The listing builds one solid part. Answer for the finished solid, in the listing's coordinates (mm). Coordinates: 2 decimals unless noted, no trailing zeros. Write each loop counter-clockwise with the first axis right and the second up, starting at its lowest first coordinate (ties: lowest second). Pieces come first, ordered by that corner, then holes.
(1) The part is cut by section A-A on z = 0. Determine the outline of the cut face in (x, y).
(2) The part is cut by section B-B on y = 10. Determine the outline of the cut face in (x, z).
(3) The part is cut by section D-D on y = 31.5. Determine the outline of the cut face in (x, z), plus the area to 3 significant figures.
(4) The part is cut by section C-C on x = 2. Determine the outline of the cut face in (y, z).
(5) Straight lines are drawn through the part: line 1 (Z direction, x = 2.6, y = 3); line 2 (Y direction, x = 1.1, z = -19); line 3 (Y direction, x = 0.65, z = -12.5). For each, find the intervals that lie inside material, in ascending order.
(6) Given P1, Ø4.5, axis at y = 40, z = -19, coming from the -X side, flat-ended and moving along its own axis, determine where the tip first touches the part or whether it passes through.
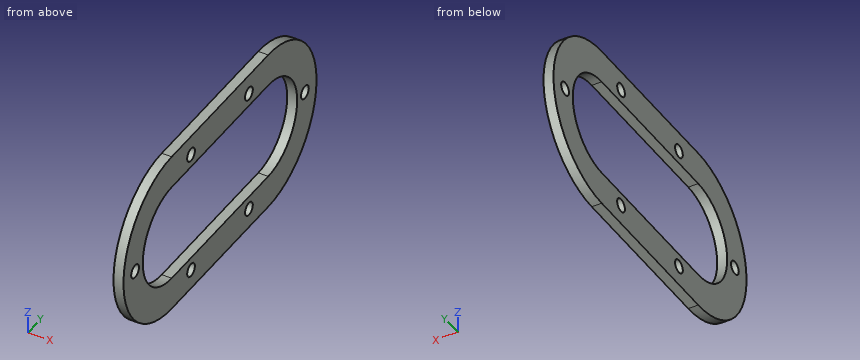
from build123d import *

# Parameters (mm, degrees)
SKETCH1_R           = 2
BOSS_EXTRUDE1_DEPTH = 3


with BuildPart() as part:
    # Sketch1 → Boss-Extrude1 (new body)
    with BuildSketch(Plane.YZ):
        with BuildLine():
            Line((0, 25), (50, 25))
            ThreePointArc((50, 25), (75, 0), (50, -25))
            Line((50, -25), (0, -25))
            ThreePointArc((0, -25), (-25, 0), (0, 25))
        make_face()
        with Locations(Location((10, 19, 0), (0, 0, 270))):
            Circle(SKETCH1_R, mode=Mode.SUBTRACT)
        with Locations(Location((40, 19, 0), (0, 0, 270))):
            Circle(SKETCH1_R, mode=Mode.SUBTRACT)
        with Locations(Location((69, 0, 0), (0, 0, 270))):
            Circle(SKETCH1_R, mode=Mode.SUBTRACT)
        with Locations(Location((-19, 0, 0), (0, 0, 270))):
            Circle(SKETCH1_R, mode=Mode.SUBTRACT)
        with Locations(Location((10, -19, 0), (0, 0, 270))):
            Circle(SKETCH1_R, mode=Mode.SUBTRACT)
        with Locations(Location((40, -19, 0), (0, 0, 270))):
            Circle(SKETCH1_R, mode=Mode.SUBTRACT)
        with BuildLine():
            Line((0, 15), (50, 15))
            ThreePointArc((50, 15), (65, 0), (50, -15))
            Line((50, -15), (0, -15))
            ThreePointArc((0, -15), (-15, 0), (0, 15))
        make_face(mode=Mode.SUBTRACT)
    extrude(amount=BOSS_EXTRUDE1_DEPTH)


solid = part.part
Model answer:
1. outline: (0, -25) - (3, -25) - (3, -21) - (0, -21) - close; (0, -17) - (3, -17) - (3, -15) - (0, -15) - close; (0, 65) - (3, 65) - (3, 67) - (0, 67) - close; (0, 71) - (3, 71) - (3, 75) - (0, 75) - close
2. outline: (0, -25) - (3, -25) - (3, -21) - (0, -21) - close; (0, -17) - (3, -17) - (3, -15) - (0, -15) - close; (0, 15) - (3, 15) - (3, 17) - (0, 17) - close; (0, 21) - (3, 21) - (3, 25) - (0, 25) - close
3. outline: (0, -25) - (3, -25) - (3, -15) - (0, -15) - close; (0, 15) - (3, 15) - (3, 25) - (0, 25) - close
3. area: 60.0 mm2
4. outline: (0, -25) - (50, -25) arc R25 ccw to (50, 25) - (0, 25) arc R25 ccw to start; hole circle Ø4 at (-19, 0); hole (0, -15) - (50, -15) arc R15 ccw to (50, 15) - (0, 15) arc R15 ccw to start; hole circle Ø4 at (10, -19); hole circle Ø4 at (10, 19); hole circle Ø4 at (40, -19); hole circle Ø4 at (40, 19); hole circle Ø4 at (69, 0)
5. line 1: z = -25 to -15, 15 to 25
5. line 2: y = -16.25 to 8, 12 to 38, 42 to 66.25
5. line 3: y = -21.65 to -8.29, 58.29 to 71.65
6. P1: stops at x = 0
